Geometry: final body of the model. Coordinates: model frame, mm. A direction names the side the tool comes from. Give positions to 0.01 mm unless a question says otherwise; leave off trailing zeros. Loops run counter-clockwise (first coordinate to the right, second up) from the corner with the lowest first, then second, coordinate; pieces in that order, holes last. Notation, with made-up numbers: (88, 37.5) -> (106, 37.5) arc R32 ccw to (106, 71.5) -> close; hole circle Ø1 at (7.5, 29.25). An arc over 180 degrees is marked (long way). Answer in a Markdown table with one row per item. Add a question column.
1) Section query C-C (y = 24). Give the number of separate pieces and of enclosed holes in the cut face, plus the area to 3 significant figures.
2) Section query B-B (z = -45). Return the cut outline in (x, y), plus the area to 3 significant figures.
3) Access query for faces 5 (the flat face through (-20, 25, -29)), 6 (the flat face through (-60, 38, -10)), 7 (the flat face through (-12, 50, -32)). Directions: +Z, -Z, +X, -X, +Y, -Y. A direction counts if a zero-diameter tool reaches every point of the face in a straight line with its end or side. Return the directions, or none.
4) Draft query along Y for faces 1 (the flat face through (-12, 48, -13)), 2 (the cylindrical face through (-59.86, 17.34, -68.475)), 3 (the flat face through (-35, 15, -10)), 4 (the flat face through (-35, 0, -8)). Return one class per face: +Y half, -Y half, draft (parallel to the pull), parting line (faces both ways), or undercut.
5) Line query: line 1 (Y direction, x = -12, z = -50); line 2 (X direction, y = 20, z = -18); line 3 (Z direction, x = -30.5, y = 10). Output: solid intervals per line, ascending. Write a range as from..to.
6) First-contact query: P1, Ø24, axis at x = -34, y = 14.5, coming from the -Z side; P2, Ø24, axis at y = 25, z = -50, coming from the +X side; P3, Ø16.5, axis at x = -14.5, y = 37, coming from the +Z side; P4, Ø4, axis at x = -8, y = 42.5, coming from the -Z side. Flat tips, straight axial feed; report the tip coordinate or a pass-through.
Autodesk Inventor part; units mm, degrees
ref_plane "YZ Plane" through (0, 0, 0) normal (1, 0, 0) x (0, 1, 0)
ref_plane "XZ Plane" through (0, 0, 0) normal (0, 1, 0) x (-1, 0, 0)
ref_plane "XY Plane" through (0, 0, 0) normal (0, 0, 1) x (1, 0, 0)
sketch "Sketch1" plane through (0, 0, 0) normal (0, 1, 0) x (-1, 0, 0)
  line L0 (0, 0) -> (70, 0)
  line L1 (70, 0) -> (70, -84.6705) construction
  line L2 (0, -84.6705) -> (0, 0) construction
  line L3 (70, 0) -> (0, 0) construction
  line L4 (0, 0) -> (0, -75)
  line L5 (0, -75) -> (20, -75)
  line L6 (20, -75) -> (20, -10)
  line L7 (20, -10) -> (50, -10)
  line L8 (50, -10) -> (50, -75)
  line L9 (50, -75) -> (70, -75)
  line L10 (70, -75) -> (70, 0)
  dimension "d0" = 70
  dimension "d1" = 20
  dimension "d2" = 30
  dimension "d3" = 20
  dimension "d4" = 10
  dimension "d20" = 65
extrude "Extrusion1" add sketch "Sketch1" along normal blind 50
sketch "Sketch2" plane through (0, 50, 0) normal (0, 1, 0) x (1, 0, 0)
  line L0 (-70, 0) -> (0, 0)
  line L1 (0, 0) -> (-70, 0)
  line L2 (-70, 0) -> (-70, 10)
  line L3 (-70, 10) -> (0, 10)
  line L4 (0, 10) -> (0, 0)
  dimension "d7" = 70
  dimension "d8" = 10
extrude "Extrusion2" cut sketch "Sketch2" against normal blind 20
fillet "Fillet1" radius 10 1 edges at (-35, 30, 0)
fillet "Fillet2" radius 25 4 edges at (-10, 50, -75) (-10, 0, -75) (-60, 0, -75) (-60, 50, -75)
chamfer "Chamfer1" distance 5 angle 45 8 edges at (0, 0, -25.0003) (0, 42.6778, -67.6778) (0, 50, -30.0003) (-70, 50, -30.0002) (-70, 7.3222, -67.6778) (-70, 0, -25.0002) (-60, 50, -10) (-10, 50, -10)
sketch "Sketch4" plane through (0, 25, -50) normal (1, 0, 0) x (0, 0, -1)
  circle A0 centre (0, 0) radius 20
  point P0 (-50, -25)
  dimension "d17" = 40
extrude "Extrusion3" cut sketch "Sketch4" against normal through all
properties part number "dhillg25_Lab2"
Evaluation:
| question | item | result |
|---|---|---|
| 1 | separate pieces | 3 |
| 1 | enclosed holes | 0 |
| 1 | area | 1,620 mm² |
| 2 | outline | (-70, 5) -> (-65, 0) -> (-50, 0) -> (-50, 5.64) -> (-70, 5.64) -> close; (-70, 44.36) -> (-50, 44.36) -> (-50, 50) -> (-65, 50) -> (-70, 45) -> close; (-20, 0) -> (-5, 0) -> (0, 5) -> (0, 5.64) -> (-20, 5.64) -> close; (-20, 44.36) -> (0, 44.36) -> (0, 45) -> (-5, 50) -> (-20, 50) -> close |
| 2 | area | 401 mm² |
| 3 | face 5 | -Z, +Y, -Y |
| 3 | face 6 | +Z, +X, -X, +Y |
| 3 | face 7 | +Z, -Z, +X, -X, +Y |
| 4 | face 1 | +Y half |
| 4 | face 2 | undercut |
| 4 | face 3 | draft |
| 4 | face 4 | -Y half |
| 5 | line 1 | 0..5, 45..50 |
| 5 | line 2 | -70..-50, -20..0 |
| 5 | line 3 | -10..0 |
| 6 | P1 | z = -10 |
| 6 | P2 | through |
| 6 | P3 | z = -5.16 |
| 6 | P4 | z = -69.62 |
